from build123d import *

# Parameters (mm, degrees)
TAGLIO_ESTRUSIONE4_START = 16
TAGLIO_ESTRUSIONE4_DEPTH = 5
TAGLIO_ESTRUSIONE5_START = 11.5
TAGLIO_ESTRUSIONE5_DEPTH = 4
SMUSSO5_SIZE             = 1


with BuildPart() as part:
    # Schizzo4 → Rivoluzione1 (revolve)
    with BuildSketch(Plane(origin=(0, 0, 0), x_dir=(0, 0, -1), z_dir=(1, 0, 0)), mode=Mode.PRIVATE) as rivoluzione1_sk:
        Polygon((0, 0), (216, 0), (216, 12.5), (194, 12.5), (194, 16), (153.5, 16), (153.5, 20), (145.5, 20), (145.5, 18.5), (102, 18.5), (102, 15), (77, 15), (77, 11.5), (0, 11.5), align=None)
    revolve(rivoluzione1_sk.sketch.rotate(Axis((0, 0, 0), (0, 0, -1)), 90), axis=Axis((0, 0, 0), (0, 0, -1)))

    # Schizzo10 → Taglia-Rivoluzione1 (revolve, cut)
    with BuildSketch(Plane(origin=(0, 0, 0), x_dir=(0, 0, -1), z_dir=(1, 0, 0)), mode=Mode.PRIVATE) as taglia_rivoluzione1_sk:
        Polygon((183.095854812, 16), (183.5, 15.3), (185.2, 15.3), (185.2, 16), align=None)
    revolve(taglia_rivoluzione1_sk.sketch.rotate(Axis((0, 0, -141.39065809), (0, 0, -1)), 90), axis=Axis((0, 0, -141.39065809), (0, 0, -1)), mode=Mode.SUBTRACT)

    # Schizzo11 → Taglia-Rivoluzione2 (revolve, cut)
    with BuildSketch(Plane(origin=(0, 0, 0), x_dir=(0, 0, -1), z_dir=(1, 0, 0)), mode=Mode.PRIVATE) as taglia_rivoluzione2_sk:
        Polygon((210.682457352, 12.5), (211, 11.95), (212.4, 11.95), (212.4, 12.5), align=None)
    revolve(taglia_rivoluzione2_sk.sketch.rotate(Axis((0, 0, -146.205163042), (0, 0, -1)), 90), axis=Axis((0, 0, -146.205163042), (0, 0, -1)), mode=Mode.SUBTRACT)

    # Schizzo12 → Taglia-Rivoluzione3 (revolve, cut)
    with BuildSketch(Plane(origin=(0, 0, 0), x_dir=(0, 0, -1), z_dir=(1, 0, 0)), mode=Mode.PRIVATE) as taglia_rivoluzione3_sk:
        Polygon((83.404145188, 15), (83, 14.3), (81.3, 14.3), (81.3, 15), align=None)
    revolve(taglia_rivoluzione3_sk.sketch.rotate(Axis((0, 0, -46.884155284), (0, 0, -1)), 90), axis=Axis((0, 0, -46.884155284), (0, 0, -1)), mode=Mode.SUBTRACT)

    # Schizzo6 → Taglio-Estrusione4 (cut)
    with BuildSketch(Plane(origin=(0, 0, 0), x_dir=(0, 0, -1), z_dir=(1, 0, 0)).offset(TAGLIO_ESTRUSIONE4_START)):
        with BuildLine():
            Line((161.5, 5), (176.5, 5))
            ThreePointArc((176.5, 5), (181.5, 0), (176.5, -5))
            Line((176.5, -5), (161.5, -5))
            ThreePointArc((161.5, -5), (156.5, 0), (161.5, 5))
        make_face()
    extrude(amount=-TAGLIO_ESTRUSIONE4_DEPTH, mode=Mode.SUBTRACT)

    # Schizzo8 → Taglio-Estrusione5 (cut)
    with BuildSketch(Plane(origin=(0, 0, 0), x_dir=(0, 0, -1), z_dir=(1, 0, 0)).offset(TAGLIO_ESTRUSIONE5_START)):
        with BuildLine():
            Line((8, 4), (22, 4))
            ThreePointArc((22, 4), (26, 0), (22, -4))
            Line((22, -4), (8, -4))
            ThreePointArc((8, -4), (4, 0), (8, 4))
        make_face()
    extrude(amount=-TAGLIO_ESTRUSIONE5_DEPTH, mode=Mode.SUBTRACT)

    # Smusso5
    smusso5_edges = [part.edges().sort_by_distance(p)[0] for p in [
        (-11.5, 0, 0),
        (-15, 0, -77),
        (-16, 0, -194),
        (-12.5, 0, -216),
    ]]
    chamfer(smusso5_edges, length=SMUSSO5_SIZE)


solid = part.part
Source: CAD feature listing. Evaluate the final solid. Frame: model axes, mm. A direction names the side the tool comes from. Give positions to 0.01 mm unless a question says otherwise; leave off trailing zeros. Order: outer loops, then holes, each group sorted by start corner. A loop starts at its lowest first (then second) coordinate and runs counter-clockwise, first axis right, second up. Notation, with made-up numbers: (-25, 87.5) -> (23, 87.5) arc R19 ccw to (23, 105.5) -> close; hole circle Ø3 at (10, 82.5). An arc over 180 degrees is marked (long way). Use a Markdown table: item, result.
1) Mould query, pull axis Z, two halves, no side actions, for faces 4 (the cylindrical face through (-3.47, 15.62, -189.05)), 5 (the cylindrical face through (-1.86, -14.18, -82.14)), 6 (the flat face through (-0.1, -15.2, -102)). Classes: +Z half, -Z half, draft (parallel to the pull), parting line (faces both ways), or undercut.
Answer list:
| item | result |
|---|---|
| face 4 | draft |
| face 5 | undercut |
| face 6 | +Z half |
2) Reachability of faces 1 (the flat face through (3.4, -12.3, -194)), 2 (the cylindrical face through (8.06, -12.65, -79.63)), 3 (the cylindrical face through (6.42, -10.08, -211.71)) from +Z, -Z, +X, -X, +Y, -Y: full face, straight path, thin tool, end or side. Return the list, or none.
Answer list:
| item | result |
|---|---|
| face 1 | -Z |
| face 2 | +Z |
| face 3 | none |
3) Section query B-B, the plane z = -173.5. Return the cut outline in (x, y).
Answer list:
| item | result |
|---|---|
| outline | (11, -5) -> (11, 5) -> (15.2, 5) arc R16 ccw (long way) to (15.2, -5) -> close |
4) Section query A-A, the plane z = -200.5. Return the cut outline in (x, y).
Answer list:
| item | result |
|---|---|
| outline | circle Ø25 at (0, 0) |
5) Contact query for flat-ended pins moving along their axis: P1, Ø20, axis at x = 2, y = 2, coming from the +Z side; P2, Ø5, axis at x = 9, z = -60.5, coming from the -Y side; P3, Ø6.5, axis at y = -0.5, z = -16, coming from the +X side; P4, Ø2, axis at x = 6, z = -59, coming from the +Y side. Output: stop coordinate, or through.
Answer list:
| item | result |
|---|---|
| P1 | z = 0 |
| P2 | y = -9.49 |
| P3 | x = 7.5 |
| P4 | y = 10.36 |
6) Ray query, line 1 along X through (y, z) = (-0.5, -154); line 2 along Z through (x, y) = (8, 17.5); line 3 along Z through (x, y) = (-1, -16). Return the intervals inside material, ascending. Write a range as [from, to].
Answer list:
| item | result |
|---|---|
| line 1 | [-15.99, 15.99] |
| line 2 | [-153.5, -145.5] |
| line 3 | [-153.5, -102] |
7) Section query C-C, the plane z = -53. Return the cut outline in (x, y).
Answer list:
| item | result |
|---|---|
| outline | circle Ø23 at (0, 0) |
